Can you work these out from the model? Positions are in its coordinate system, mm. A direction names the side the tool comes from. Coordinates: 2 decimals unless noted, no trailing zeros. Order: outer loops, then holes, each group sorted by start corner. A loop starts at its lowest first (then second) coordinate and runs counter-clockwise, first axis right, second up. Notation, with made-up numbers: (24.5, -12) -> (50.5, -12) arc R8 ccw to (50.5, 2) -> close; hole circle Ø5 at (-7, 29). An arc over 180 degrees is marked (long way). Answer as CSV lines item,"result".
from build123d import *

# Parameters (mm, degrees)
BOSS_EXTRUDE1_DEPTH = 2.54
BOSS_EXTRUDE2_DEPTH = 1.778


with BuildPart() as part:
    # Sketch1 → Boss-Extrude1 (new body)
    with BuildSketch(Plane(origin=(0, 0, 0), x_dir=(1, 0, 0), z_dir=(0, 1, 0))):
        with BuildLine():
            Line((0, 15.24), (0, 0))
            Line((0, 0), (7.112, 0))
            Line((7.112, 0), (7.112, 15.24))
            ThreePointArc((7.112, 15.24), (3.556, 11.684), (0, 15.24))
        make_face()
    extrude(amount=BOSS_EXTRUDE1_DEPTH)

    # Sketch2 → Boss-Extrude2 (add)
    with BuildSketch(Plane.XZ):
        Polygon((0, 0), (3.556, 0), (0, -11.684), align=None)
    extrude(amount=BOSS_EXTRUDE2_DEPTH)


solid = part.part
Q1. Imagine slicing it at C-C (x = 6.75). List the corners of the cut face in (y, z) for me, and give its area (3 significant figures).
Solution:
outline,"(0, -13.68) -> (2.54, -13.68) -> (2.54, 0) -> (0, 0) -> close"
area,"34.7 mm2"
Q2. Which directions (+Z, -Z, +X, -X, +Y, -Y) give clear straight access to the entire face, cutting with the end or side of a thin tool? Please do faces 4 (the flat face through (4, 0, -8)), 5 (the flat face through (0, 0, -8)).
Solution:
face 4,"-Z, +X, -Y"
face 5,"+Z, -Z, -X, +Y, -Y"
Q3. For P1, Ø1, axis at x = 1.5, y = 2, coming from the +Z side; P2, Ø1, axis at x = 1.5, z = -11, coming from the -Y side, each with a flat end and sliding along its axis, tell me the tip position at first contact or that it passes through.
Solution:
P1,"z = 0"
P2,"y = 0"
Q4. Imagine slicing it at A-A (z = -2.5). List the corners of the cut face in (x, y) for me, and give its area (3 significant figures).
Solution:
outline,"(0, -1.78) -> (2.8, -1.78) -> (2.8, 0) -> (7.11, 0) -> (7.11, 2.54) -> (0, 2.54) -> close"
area,"23.0 mm2"
Q5. If I drill on line 1 (Y direction, x = 4.25, z = -9.25); line 2 (Z direction, x = 6.25, y = 2.25); line 3 (Z direction, x = 5.5, y = 1.55), over which ranges is the centre line in solid material (lowest first)?
Solution:
line 1,"0 to 2.54"
line 2,"-12.92 to 0"
line 3,"-12.26 to 0"
Q6. Imagine slicing it at D-D (z = -9.5). List the corners of the cut face in (x, y) for me, and give its area (3 significant figures).
Solution:
outline,"(0, -1.78) -> (0.66, -1.78) -> (0.66, 0) -> (7.11, 0) -> (7.11, 2.54) -> (0, 2.54) -> close"
area,"19.2 mm2"
Q7. We'd pull the mould along X, two halves only. Please class faces 1 (the cylindrical face through (3.634, 1.252, -11.685)), 2 (the flat face through (3, 1, 0)), 3 (the flat face through (7.112, 1, -8)): pulls with the +X half, pulls with the -X half, needs draft (parallel to the pull), parting line crosses it, or undercut.
Solution:
face 1,"undercut"
face 2,"needs draft"
face 3,"pulls with the +X half"
